Build history of the part. All positions in model axes, mm. Face numbers are marked on the shaded views. A direction names the side the tool comes from. Coordinates: 2 decimals unless noted, no trailing zeros. Order: outer loops, then holes, each group sorted by start corner. A loop starts at its lowest first (then second) coordinate and runs counter-clockwise, first axis right, second up. Notation, with made-up numbers: (-28, 48) -> (0, 48) arc R19 cw to (0, 70) -> close; hole circle Ø10 at (-21, 76.5). An arc over 180 degrees is marked (long way). Write each question's results on one line, items separated by ' | '.
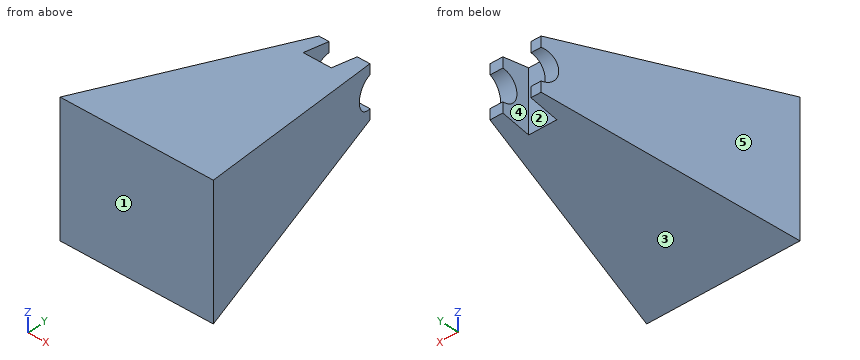
from build123d import *

# Parameters (mm, degrees)
BOSS_EXTRUDE1_DEPTH     = 65.000000048
CUT_EXTRUDE1_DEPTH      = 39.1
CUT_EXTRUDE1_DEPTH_BACK = 39.1
SKETCH4_W               = 13.97
SKETCH4_H               = 13.97
CUT_EXTRUDE2_DEPTH      = 1
CUT_EXTRUDE2_DEPTH_BACK = 66.000000048
CUT_EXTRUDE4_DEPTH      = 39.1
CUT_EXTRUDE4_DEPTH_BACK = 39.1


with BuildPart() as part:
    # Sketch2 → Boss-Extrude1 (new body)
    with BuildSketch(Plane.XY):
        Polygon((-38.1, -56.007), (-12.7, 56.007), (12.7, 56.007), (38.1, -56.007), align=None)
    extrude(amount=-BOSS_EXTRUDE1_DEPTH)

    # Sketch3 → Cut-Extrude1 (cut, two sides)
    with BuildSketch(Plane(origin=(0, 0, 0), x_dir=(0, 0, -1), z_dir=(1, 0, 0))) as cut_extrude1_sk:
        Polygon((0, -56.007), (19.800000024, 56.007), (0, 56.007), align=None)
        Polygon((65.000000048, -56.007), (45.200000024, 56.007), (65.000000048, 56.007), align=None)
    extrude(amount=CUT_EXTRUDE1_DEPTH, mode=Mode.SUBTRACT)
    extrude(cut_extrude1_sk.sketch, amount=-CUT_EXTRUDE1_DEPTH_BACK, mode=Mode.SUBTRACT)

    # Sketch4 → Cut-Extrude2 (cut, two sides)
    with BuildSketch(Plane.XY) as cut_extrude2_sk:
        with Locations((-0.635, 49.022)):
            Rectangle(SKETCH4_W, SKETCH4_H)
    extrude(amount=CUT_EXTRUDE2_DEPTH, mode=Mode.SUBTRACT)
    extrude(cut_extrude2_sk.sketch, amount=-CUT_EXTRUDE2_DEPTH_BACK, mode=Mode.SUBTRACT)

    # Sketch5 → Cut-Extrude4 (cut, two sides)
    with BuildSketch(Plane(origin=(0, 0, 0), x_dir=(0, 0, -1), z_dir=(1, 0, 0))) as cut_extrude4_sk:
        with BuildLine():
            Line((40.120000024, 56.007), (24.880000024, 56.007))
            ThreePointArc((24.880000024, 56.007), (32.500000024, 48.387), (40.120000024, 56.007))
        make_face()
    extrude(amount=CUT_EXTRUDE4_DEPTH, mode=Mode.SUBTRACT)
    extrude(cut_extrude4_sk.sketch, amount=-CUT_EXTRUDE4_DEPTH_BACK, mode=Mode.SUBTRACT)


solid = part.part
Item 1: Drill centre lines: line 1 (X direction, y = 47, z = -42.5); line 2 (Y direction, x = -3, z = -26.5); line 3 (X direction, y = 39.5, z = -22). Where is each one in solid material? Low to high. Write a range as from..to.
Answer:
line 1: x = -14.74..-7.62, 6.35..14.74 | line 2: y = -56.01..42.04 | line 3: x = -16.44..16.44
Item 2: Tool access for the marked faces 1 and 2: list every direction of +Z, -Z, +X, -X, +Y, -Y with a clear straight run to the whole face (end or side of a thin tool).
Answer:
face 1: +Z, -Z, +X, -X, -Y | face 2: +Z, -Z, +Y
Item 3: Pin check, flat tips, straight feed: pin 1 (15.5 mm diameter, centred on x = -0.5, z = -25.5, fed in from +Y); pin 2 (1.5 mm diameter, centred on x = -14.5, y = -26, fed in from -Z); pin 3 (6 mm diameter, centred on y = 2.5, z = -8.5, fed in from -X); pin 4 (6 mm diameter, centred on y = -12.5, z = -15.5, fed in from -X). Stop position of each tip, or through.
Answer:
pin 1: stops at y = 56.01 | pin 2: stops at z = -59.83 | pin 3: stops at x = -25.44 | pin 4: stops at x = -28.91
Item 4: Slice it at A-A, the plane z = -32.5. List the corners of the cut face in (x, y), and give its area (3 significant figures).
Answer:
outline: (-38.1, -56.01) -> (38.1, -56.01) -> (14.43, 48.39) -> (6.35, 48.39) -> (6.35, 42.04) -> (-7.62, 42.04) -> (-7.62, 48.39) -> (-14.43, 48.39) -> close | area: 5,390 mm^2
Item 5: Slice it at B-B, the plane x = -11. List the corners of the cut face in (y, z).
Answer:
outline: (-56.01, -65) -> (56.01, -45.2) -> (56.01, -40.12) arc R7.62 cw to (56.01, -24.88) -> (56.01, -19.8) -> (-56.01, 0) -> close
Item 6: Slice it at C-C, the plane z = -41.5. List the corners of the cut face in (x, y), and give its area (3 significant figures).
Answer:
outline: (-38.1, -56.01) -> (38.1, -56.01) -> (12.7, 56.01) -> (6.35, 56.01) -> (6.35, 42.04) -> (-7.62, 42.04) -> (-7.62, 56.01) -> (-12.7, 56.01) -> close | area: 5,500 mm^2
Item 7: Pull direction X, two halves, no side cores. Call the marked faces 3, 4 and 5: released by +X, released by -X, zero draft, split by the parting line, or undercut.
Answer:
face 3: zero draft | face 4: undercut | face 5: released by -X
Item 8: Slice it at D-D, the plane y = 34.5. List the corners of the cut face in (x, z), and give its area (3 significant figures).
Answer:
outline: (-17.58, -49) -> (17.58, -49) -> (17.58, -16) -> (-17.58, -16) -> close | area: 1,160 mm^2
